from build123d import *

# Parameters (mm, degrees)
F1_DEPTH = 2
F3_DEPTH = 2.001


with BuildPart() as f1:
    # F0 (on Front) → F1 (new body)
    with BuildSketch(Plane.XZ):
        with BuildLine():
            Line((4.4, 8), (4.4, 5))
            Line((4.4, 5), (2.8, 5))
            Line((2.8, 5), (2.8, 8))
            Line((2.8, 8), (-2.8, 8))
            Line((-2.8, 8), (-2.8, 5))
            Line((-2.8, 5), (-4.4, 5))
            Line((-4.4, 5), (-4.4, 8))
            Line((-4.4, 8), (-5.5, 8))
            Line((-5.5, 8), (-5.5, 5))
            Line((-5.5, 5), (-5.5, 0.366807))
            ThreePointArc((-5.5, 0.366807), (-6.37868, -1.754513), (-8.5, -2.633193))
            Line((-8.5, -2.633193), (-8.368722, -2.633193))
            ThreePointArc((-8.368722, -2.633193), (-10.735529, -5), (-8.368722, -7.366807))
            Line((-8.368722, -7.366807), (8.368722, -7.366807))
            ThreePointArc((8.368722, -7.366807), (10.735529, -5), (8.368722, -2.633193))
            Line((8.368722, -2.633193), (8.5, -2.633193))
            ThreePointArc((8.5, -2.633193), (6.37868, -1.754513), (5.5, 0.366807))
            Line((5.5, 0.366807), (5.5, 5))
            Line((5.5, 5), (5.5, 8))
            Line((5.5, 8), (4.4, 8))
        make_face()
    extrude(amount=F1_DEPTH)

    # F2 (on face) → F3 (cut, through all)
    with BuildSketch(Plane.XZ.offset(2)):
        with BuildLine():
            ThreePointArc((5.203029, -3.108616), (4.076106, -1.909689), (3.751051, -0.296703))
            ThreePointArc((3.751051, -0.296703), (0, 3.762767), (-3.751051, -0.296703))
            ThreePointArc((-3.751051, -0.296703), (-4.076106, -1.909689), (-5.203029, -3.108616))
            Line((-5.203029, -3.108616), (-5.605626, -3.349153))
            ThreePointArc((-5.605626, -3.349153), (-6.760531, -3.749147), (-7.979135, -3.655299))
            ThreePointArc((-7.979135, -3.655299), (-9.759296, -4.837816), (-8.299049, -6.398265))
            Line((-8.299049, -6.398265), (8.368576, -6.4))
            ThreePointArc((8.368576, -6.4), (9.754839, -4.803326), (7.979135, -3.655299))
            ThreePointArc((7.979135, -3.655299), (6.760531, -3.749147), (5.605626, -3.349153))
            Line((5.605626, -3.349153), (5.203029, -3.108616))
        make_face()
    extrude(amount=-F3_DEPTH, mode=Mode.SUBTRACT)


solid = f1.part
Check sheet for the modelled part. Datum: model origin and axes. Units: mm. A direction names the side the tool comes from. Round coordinates to 2 decimals unless told otherwise and drop trailing zeros. Loops run counter-clockwise (first coordinate to the right, second up) from the corner with the lowest first, then second, coordinate; pieces in that order, holes last. Notation, with made-up numbers: M 46.25,-5.5 L 92.25,-5.5 A29 cw 92.25,18.5 Z; hole C -34,59 d6. An arc over 180 degrees is marked long. One line per question, with ' | ' between items. Start each with the question number.
Item 1: Section check B-B (x = 0). Record the boundary of the cut face in (y, z).
Item 2: Scan lines: probe 1 along X at (y, z) = (-1, 7); probe 2 along X at (y, z) = (-1.3, -5); probe 3 along X at (y, z) = (-0.7, -1). Record each from-to range of solid material in increasing order.
Item 3: Section check C-C (z = 5.25). Record the boundary of the cut face in (x, y).
Item 4: Section check D-D (y = -0.55). Record the boundary of the cut face in (x, z), and give its area (3 significant figures).
Item 5: Section check A-A (z = -5). Record the boundary of the cut face in (x, y).
Item 6: Set-up check for faces 1 (the face through (-6.743, -1.014, -3.747)), 2 (the face through (0, -2, 4)), 3 (the face through (4.4, -1, 7)): record each of +Z, -Z, +X, -X, +Y, -Y from which the full face is reachable in a straight line by a thin tool's end or side.
Item 7: Gauge pin test, flat ends, axial feed: pin 1 Ø6 at (x, z) = (1, 0) entering from -Y; pin 2 Ø0.8 at (x, y) = (3.5, -1.5) entering from +Z; pin 3 Ø1 at (y, z) = (-0.5, 6.5) entering from +X. Record the tip position at first contact, or that the pin passes through.
Item 8: Release check for a two-part mould opening along X. For faces 4 (the face through (9.76, -1.01, -4.84)), 5 (the face through (-6.355, -0.986, -1.731)), 6 (the face through (0, 0, 4)), 7 (the face through (-2.8, -1, 7)) record: released by +X, released by -X, zero draft, split by the parting line, or undercut.
Worked out:
1) outline: M -2,-7.37 L 0,-7.37 L 0,-6.4 L -2,-6.4 Z; M -2,3.76 L 0,3.76 L 0,8 L -2,8 Z
2) probe 1: -5.5 to -4.4, -2.8 to 2.8, 4.4 to 5.5 | probe 2: -10.74 to -9.77, 9.77 to 10.74 | probe 3: -5.83 to -3.78, 3.78 to 5.83
3) outline: M -5.5,-2 L -4.4,-2 L -4.4,0 L -5.5,0 Z; M -2.8,-2 L 2.8,-2 L 2.8,0 L -2.8,0 Z; M 4.4,-2 L 5.5,-2 L 5.5,0 L 4.4,0 Z
4) outline: M -8.5,-2.63 L -8.37,-2.63 A2.37 ccw -8.37,-7.37 L 8.37,-7.37 A2.37 ccw 8.37,-2.63 L 8.5,-2.63 A3 cw 5.5,0.37 L 5.5,8 L 4.4,8 L 4.4,5 L 2.8,5 L 2.8,8 L -2.8,8 L -2.8,5 L -4.4,5 L -4.4,8 L -5.5,8 L -5.5,0.37 A3 cw Z; hole M -8.3,-6.4 L 8.37,-6.4 A1.4 ccw long 7.98,-3.66 A3 cw 5.61,-3.35 L 5.2,-3.11 A3 cw 3.75,-0.3 A3.76 ccw long -3.75,-0.3 A3 cw -5.2,-3.11 L -5.61,-3.35 A3 cw -7.98,-3.66 A1.4 ccw long Z | area: 102 mm^2
5) outline: M -10.74,-2 L -9.77,-2 L -9.77,0 L -10.74,0 Z; M 9.77,-2 L 10.74,-2 L 10.74,0 L 9.77,0 Z
6) face 1: +Y, -Y | face 2: +Z, -Z, +X, -X, -Y | face 3: +Z, +Y, -Y
7) pin 1: y = -2 | pin 2: z = 5 | pin 3: x = 5.5
8) face 4: undercut | face 5: released by -X | face 6: zero draft | face 7: undercut
